```python
from build123d import *

# Parameters (mm, degrees)
SKETCH1_W           = 300
SKETCH1_H           = 300
BOSS_EXTRUDE1_DEPTH = 20
FILLET1_R           = 10
SKETCH2_R           = 16.222477604
BOSS_EXTRUDE2_DEPTH = 10


with BuildPart() as part:
    # Sketch1 → Boss-Extrude1 (new body)
    with BuildSketch(Plane(origin=(0, 0, 0), x_dir=(1, 0, 0), z_dir=(0, 1, 0))):
        Rectangle(SKETCH1_W, SKETCH1_H)
    extrude(amount=BOSS_EXTRUDE1_DEPTH)

    # Fillet1
    fillet1_edges = [part.edges().sort_by_distance(p)[0] for p in [
        (150, 10, 150),
        (-150, 10, 150),
        (-150, 10, -150),
        (150, 10, -150),
    ]]
    fillet(fillet1_edges, radius=FILLET1_R)

    # Sketch2 → Boss-Extrude2 (add)
    with BuildSketch(Plane(origin=(0, 20, 0), x_dir=(1, 0, 0), z_dir=(0, 1, 0))):
        Circle(SKETCH2_R)
    extrude(amount=BOSS_EXTRUDE2_DEPTH)


solid = part.part
```
Geometry check sheet. Reference: the model listing, model coordinates, mm. A direction names the side the tool comes from. Coordinates: 2 decimals unless noted, no trailing zeros. Order: outer loops, then holes, each group sorted by start corner. A loop starts at its lowest first (then second) coordinate and runs counter-clockwise, first axis right, second up.
Item 1: Depth check by flat-ended pin: pin 1 (6 mm diameter, centred on x = -114, z = -94.5, fed in from +Y). Enter the tip coordinate at first touch or a pass-through.
Item 2: Section check D-D (x = -57.5). Enter the section's corners in (y, z), plus the area to 3 significant figures.
Item 3: Tool access check on faces 1 (the cylindrical face through (-3.517, 24.93, 15.837)), 2 (the flat face through (0, 30, 0)). Record the directions out of +Z, -Z, +X, -X, +Y, -Y that give a thin tool (end or side, any length) a straight path to the whole face; none if there is none.
Item 4: Section check B-B (z = 0). Enter the section's corners in (x, y), plus the area to 3 significant figures.
Item 5: Section check C-C (y = 24.5). Enter the section's corners in (x, z), plus the area to 3 significant figures.
Item 6: Scan lines: line 1 along Y through (x, z) = (30, 86); line 2 along Z through (x, y) = (1, 25.75). Record each from-to range of solid material in increasing order.
Item 7: Section check A-A (x = 0). Enter the section's corners in (y, z), plus the area to 3 significant figures.
Check sheet entries:
1. pin 1: stops at y = 20
2. outline: (0, -150) - (20, -150) - (20, 150) - (0, 150) - close
2. area: 6,000 mm2
3. face 1: +Y
3. face 2: +Z, -Z, +X, -X, +Y
4. outline: (-150, 0) - (150, 0) - (150, 20) - (16.22, 20) - (16.22, 30) - (-16.22, 30) - (-16.22, 20) - (-150, 20) - close
4. area: 6,320 mm2
5. outline: circle Ø32.44 at (0, 0)
5. area: 827 mm2
6. line 1: y = 0 to 20
6. line 2: z = -16.19 to 16.19
7. outline: (0, -150) - (20, -150) - (20, -16.22) - (30, -16.22) - (30, 16.22) - (20, 16.22) - (20, 150) - (0, 150) - close
7. area: 6,320 mm2
